Can you work these out from the model? Positions are in its coordinate system, mm. A direction names the side the tool comes from. Give positions to 0.01 mm unless a question says otherwise; leave off trailing zeros. Loops run counter-clockwise (first coordinate to the right, second up) from the corner with the lowest first, then second, coordinate; pieces in that order, holes last. Notation, with made-up numbers: (48, 83.5) - (58, 83.5) arc R19 ccw to (58, 91.5) - close; hole circle Ø7 at (11.5, -18.5). An arc over 180 degrees is marked (long way). Answer as a JSON object with one key per item and string values. Group by question number.
Item 1: Suppose I cut it at A-A on z = -13. Write out the boundary of the cut face in (x, y), and give its area (3 significant figures).
Item 2: Suppose I cut it at C-C on z = 20.5. Write out the boundary of the cut face in (x, y), and give its area (3 significant figures).
Item 3: Which directions (+Z, -Z, +X, -X, +Y, -Y) give clear straight access to the entire face, cutting with the end or side of a thin tool? Please do faces 5 (the flat face through (74.1, 47.58, -2.33)), 6 (the flat face through (17, 10, -1)), 7 (the flat face through (58.99, 55.92, 1.52)), 8 (the cylindrical face through (29.24, 5.3, 3.65)).
Item 4: Please list where these lines run through material, in increasing order: L1, parallel to X at y = 7, z = 0; L2, parallel to Z at x = 0, y = 7; L3, parallel to Z at x = 44.5, y = 37.5.
Item 5: Suppose I cut it at D-D on y = 28.5. Write out the boundary of the cut face in (x, z), and give its area (3 significant figures).
Item 6: Will these pins go through, and if not, where does the flat tip stop? pin 1 (19 mm diameter, centred on x = 34, z = 0, fed in from +Y); pin 2 (10 mm diameter, centred on x = 24, y = 45, fed in from +Z); pin 3 (8 mm diameter, centred on x = 11.5, y = 4, fed in from +Z).
Item 7: Thinking about a two-plate mould opening in Z: for faces 1 (the cylindrical face through (62.216, 59.88, 26.733)), 2 (the flat face through (47, 5, -8)), 3 (the flat face through (34, 0.475, 0)), 4 (the flat face through (33, 30, -25)), which applies, pulls with the +Z half, pulls with the -Z half, needs draft (parallel to the pull), parting line crosses it, or undercut?
Item 8: Suppose I cut it at B-B on x = -3. Write out the boundary of the cut face in (y, z) (3 decimals), and give its area (3 significant figures).
Autodesk Inventor part; units mm, degrees
ref_plane "YZ Plane" through (0, 0, 0) normal (1, 0, 0) x (0, 1, 0)
ref_plane "XZ Plane" through (0, 0, 0) normal (0, 1, 0) x (-1, 0, 0)
ref_plane "XY Plane" through (0, 0, 0) normal (0, 0, 1) x (1, 0, 0)
sketch "Sketch1" plane through (0, 0, 0) normal (0, 1, 0) x (-1, 0, 0)
  arc A0 (-34, 13) -> (-47, 0) centre (-34, 0) ccw
  arc A1 (13, 0) -> (0, 13) centre (0, 0) ccw
  line L0 (0, 13) -> (-34, 13)
  line L1 (13, 0) -> (13, -25)
  line L2 (13, -25) -> (-47, -25)
  line L3 (-47, -25) -> (-47, 0)
  dimension "d25" = 60
  dimension "d26" = 13
  dimension "d27" = 13
  dimension "d28" = 25
extrude "Extrusion1" add sketch "Sketch1" along normal blind 10
sketch "Sketch2" plane through (0, 10, 0) normal (0, 1, 0) x (1, 0, 0)
  arc A0 (-13, 0) -> (0, -13) centre (0, 0) ccw
  arc A1 (34, -13) -> (47, 0) centre (34, 0) ccw
  circle A2 centre (0, 0) radius 6
  circle A3 centre (34, 0) radius 6
  dimension "d29" = 12
extrude "Extrusion2" cut sketch "Sketch2" against normal blind 9.525
sketch "Sketch3" plane through (47, 0, -25) normal (0, 0, -1) x (-1, 0, 0)
  line L0 (0, 10) -> (60, 10)
  line L1 (0, 0) -> (0, 10)
  line L2 (-19.6162, 62.4195) -> (-7.3912, 75.0789)
  line L3 (-19.6162, 62.4195) -> (-30.6439, 51)
  line L4 (-30.6439, 51) -> (0, 0)
  line L5 (-7.3912, 75.0789) -> (60, 10)
  line L6 (0, 0) -> (0, 10)
  line L7 (60, 10) -> (0, 10)
  point P0 (47, 0)
  dimension "d30" = 44
  dimension "d31" = 90
  dimension "d32" = 51
  dimension "d33" = 105
extrude "Extrusion3" add sketch "Sketch3" against normal blind 10
sketch "Sketch4" plane through (54.3912, 75.0789, -25) normal (0.7193398, 0.6946584, 0) x (-0.6946584, 0.7193398, 0)
  line L0 (0, 0) -> (-33.4736, 0)
  line L1 (0, 0) -> (0, 10)
  line L2 (-33.4736, 10) -> (0, 10)
  line L3 (-33.4736, 0) -> (-33.4736, 10)
  arc A0 (0, 35) -> (-33.4736, 35) centre (-16.7368, 35) ccw
  line L4 (-33.4736, 35) -> (-33.4736, 0)
  line L5 (-33.4736, 0) -> (0, 0)
  line L6 (0, 0) -> (0, 35)
  point P0 (-16.224, 25)
  dimension "d34" = 35
extrude "Extrusion4" add sketch "Sketch4" against normal blind 10 contours L2 L4 A0 L6
hole "구멍1" at (66.0175, 63.0394, 10) direction (-0.7193398, -0.6946584, 0) diameter 15 end up to surface
properties part number "스터디캐드캠 - 3D 모델링 연습도면 540"
Worked out:
{
 "1": {"outline": "(-13, 0) - (47, 0) - (47, 10) - (-13, 10) - close; (47.2, 68.13) - (70.45, 44.05) - (77.64, 51) - (54.39, 75.08) - close", "area": "935 mm2"},
 "2": {"outline": "(49.77, 65.47) - (67.88, 46.72) - (75.07, 53.66) - (56.96, 72.41) - close", "area": "261 mm2"},
 "3": {"face 5": "+Z, +X, -Y", "face 6": "+Z, +X, -X, +Y", "face 7": "+Z, -X, -Y", "face 8": "+Y"},
 "4": {"L1": "x = -13 to -6, 6 to 28, 40 to 47", "L2": "z = -25 to -6, 6 to 13", "L3": "z = -25 to -15"},
 "5": {"outline": "(6.16, -25) - (64.12, -25) - (64.12, -15) - (6.16, -15) - close", "area": "580 mm2"},
 "6": {"pin 1": "stops at y = 10", "pin 2": "stops at z = -15", "pin 3": "stops at z = 13"},
 "7": {"face 1": "pulls with the +Z half", "face 2": "needs draft", "face 3": "undercut", "face 4": "pulls with the -Z half"},
 "8": {"outline": "(0, -25) - (19.657, -25) - (19.657, -15) - (10, -15) - (10, -5.196) - (0.475, -5.196) - (0.475, 5.196) - (10, 5.196) - (10, 12.649) - (0, 12.649) - close", "area": "374 mm2"}
}
